Part print with two shaded views. Sizes in mm from the minimum x, y, z corner. A direction names the side the tool comes from. Give positions to 0.01 mm unless a question says otherwise; leave off trailing zeros. Order: outer loops, then holes, each group sorted by start corner. A loop starts at its lowest first (then second) coordinate and runs counter-clockwise, first axis right, second up. Notation, with made-up numbers: M 63,42 L 101,42 A24 ccw 101,64 Z; hole C 77,70.25 d3. An arc over 180 degrees is marked long. Return JSON: item names as keys, results as strings. Group by question number.
1. Slice it at C-C on y = 41.5. List the corners of the cut face in (x, z), then the cut area to 3 significant figures.
2. Slice it at D-D on x = 25. List the corners of the cut face in (y, z), then the cut area to 3 significant figures.
3. Two-plate mould, pull along Y, no slides. Class the marked faces 4, 5, 6 and 7: released by +Y, released by -Y, zero draft, split by the parting line, or undercut.
4. Pin check, flat tips, straight feed: pin 1 (5.5 mm diameter, centred on y = 62, z = 9.5, fed in from -X); pin 2 (12 mm diameter, centred on x = 25, y = 26.5, fed in from +Z); pin 3 (10 mm diameter, centred on y = 61.5, z = 43, fed in from +X); pin 4 (6 mm diameter, centred on y = 61.5, z = 43, fed in from -X). Stop position of each tip, or through.
5. Slice it at A-A on y = 12.5. List the corners of the cut face in (x, z).
6. Slice it at B-B on z = 20.5. List the corners of the cut face in (x, y), then the cut area to 3 significant figures.
7. Wall check: probe 1 along Z at (x, y) = (2, 12); probe 2 along Y at (x, z) = (7.55, 8); probe 3 along Y at (x, z) = (36.5, 25). Give the ranges that are in metal, low to high. Write a range as [from, to].
8. 3-axis set-ups, long thin cutter, end or side, ignore diameter. For the marked faces 1, 2 and 3: which of +Z, -Z, +X, -X, +Y, -Y reach the whole face in a straight line?
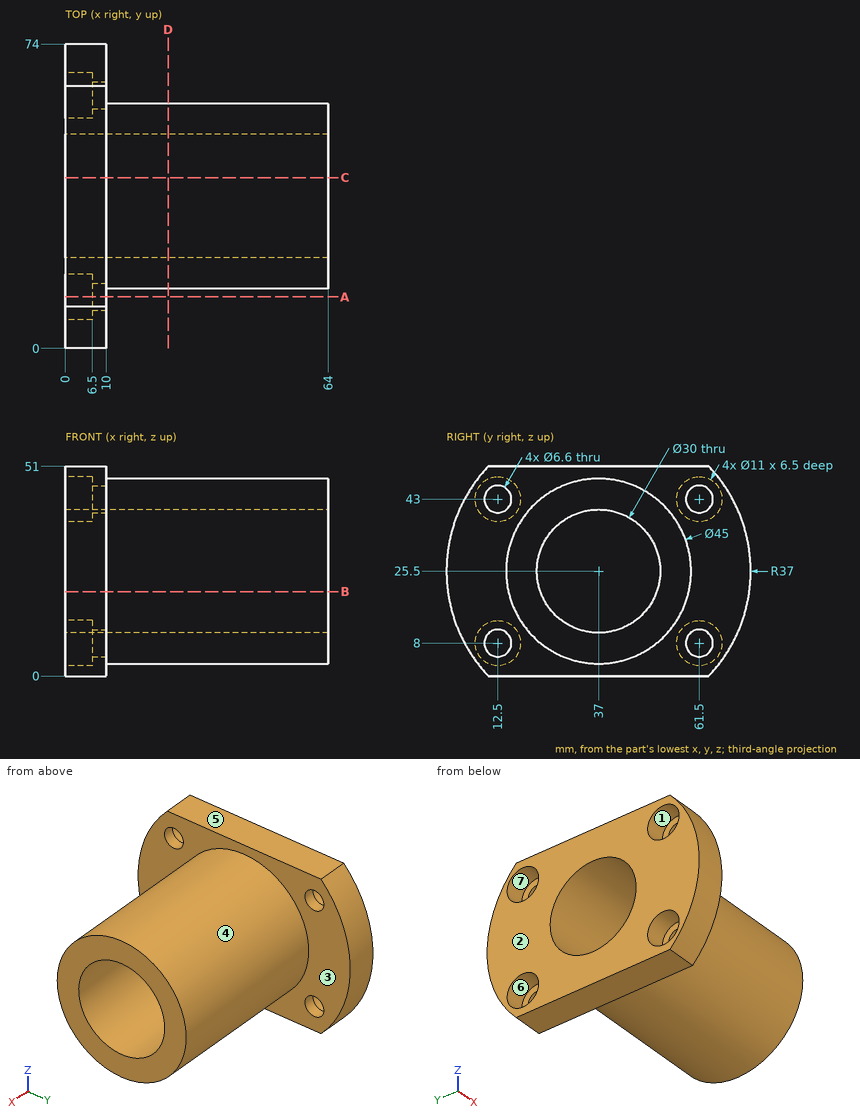
Result:
{
 "1": {"outline": "M 0,0 L 10,0 L 10,3.45 L 64,3.45 L 64,11.19 L 0,11.19 Z; M 0,39.81 L 64,39.81 L 64,47.55 L 10,47.55 L 10,51 L 0,51 Z", "area": "1,060 mm2"},
 "2": {"outline": "C 37,25.5 d45; hole C 37,25.5 d30", "area": "884 mm2"},
 "3": {"face 4": "split by the parting line", "face 5": "zero draft", "face 6": "undercut", "face 7": "undercut"},
 "4": {"pin 1": "stops at x = 6.5", "pin 2": "stops at z = 47.55", "pin 3": "stops at x = 10", "pin 4": "passes through"},
 "5": {"outline": "M 0,0 L 10,0 L 10,4.7 L 6.5,4.7 L 6.5,2.5 L 0,2.5 Z; M 0,13.5 L 6.5,13.5 L 6.5,11.3 L 10,11.3 L 10,39.7 L 6.5,39.7 L 6.5,37.5 L 0,37.5 Z; M 0,48.5 L 6.5,48.5 L 6.5,46.3 L 10,46.3 L 10,51 L 0,51 Z"},
 "6": {"outline": "M 0,0.34 L 10,0.34 L 10,15.06 L 64,15.06 L 64,22.86 L 0,22.86 Z; M 0,51.14 L 64,51.14 L 64,58.94 L 10,58.94 L 10,73.66 L 0,73.66 Z", "area": "1,290 mm2"},
 "7": {"probe 1": "z = [0, 2.52], [13.48, 37.52], [48.48, 51]", "probe 2": "y = [4.4, 9.2], [15.8, 58.2], [64.8, 69.6]", "probe 3": "y = [14.51, 22.01], [51.99, 59.49]"},
 "8": {"face 1": "-X", "face 2": "+Z, -Z, -X, +Y, -Y", "face 3": "+X"}
}
